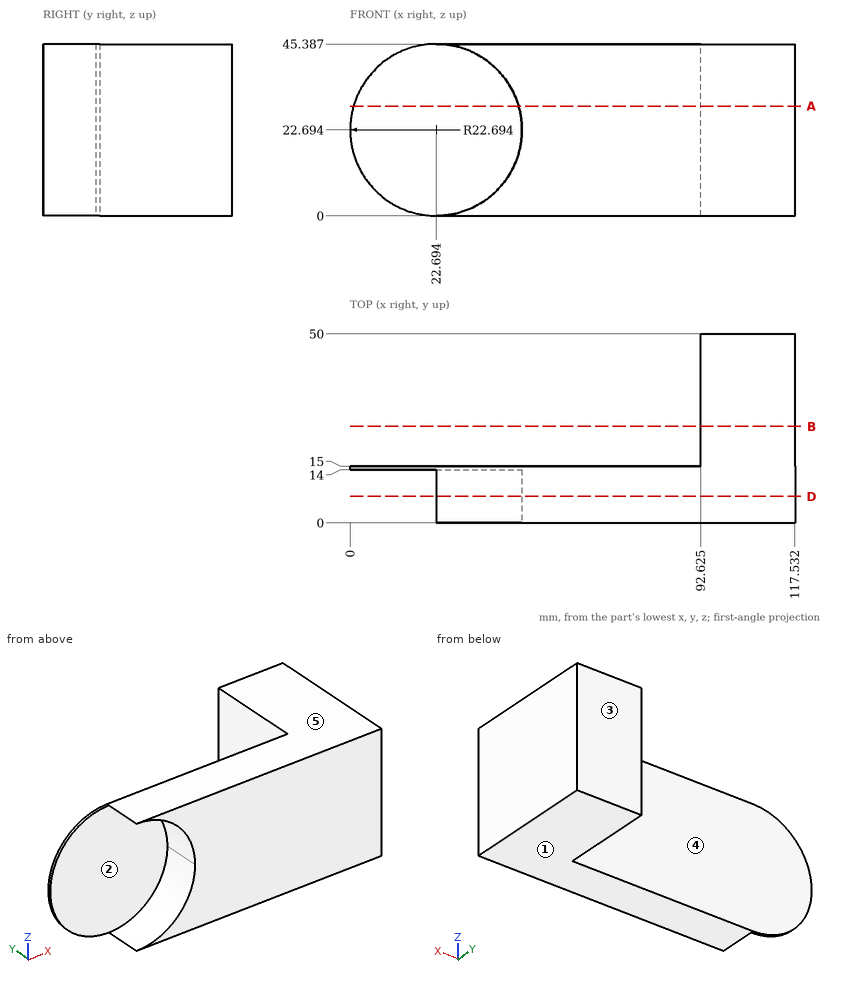
Here's the drawing with two shaded views (mm, measured from the low corner). I have some questions. A direction names the side the tool comes from. Round coordinates to 2 decimals unless told otherwise and drop trailing zeros. Order: outer loops, then holes, each group sorted by start corner. A loop starts at its lowest first (then second) coordinate and runs counter-clockwise, first axis right, second up. Notation, with made-up numbers: (29.5, 15) -> (62.5, 15) arc R20 ccw to (62.5, 20) -> close; hole circle Ø3 at (89, -26). An arc over 180 degrees is marked (long way). Return JSON: item names as keys, results as strings.
Q1. If we section it at B-B on y = 25.5: List the corners of the cut face in (x, z) for me (1 decimal), plus the area to 3 significant figures.
Filled sheet:
{"outline": "(92.6, 0) -> (117.5, 0) -> (117.5, 45.4) -> (92.6, 45.4) -> close", "area": "1,130 mm^2"}
Q2. For pin 1 Ø4 at (y, z) = (39.5, 18.5) entering from -X (3 decimals); pin 2 Ø4 at (x, z) = (44, 9.5) entering from +Y; pin 3 Ø22.5 at (x, z) = (24, 29) entering from -Y; pin 4 Ø6 at (x, y) = (89.5, 33) entering from -Z, each with a flat end and sliding along its axis, tell me the tip position at first contact or that it passes through.
Filled sheet:
{"pin 1": "stops at x = 92.625", "pin 2": "stops at y = 15", "pin 3": "stops at y = 14", "pin 4": "passes through"}
Q3. If we mould it in two halves opening along Z, with no side actions, what happens to the marked faces 1, 2 and 3? For each: released by +Z, released by -Z, zero draft, split by the parting line, or undercut.
Filled sheet:
{"face 1": "released by -Z", "face 2": "undercut", "face 3": "zero draft"}
Q4. I need wall thicknesses on line 1 along X through (y, z) = (40, 5) (1 decimal); line 2 along Y through (x, z) = (72, 32); line 3 along X through (y, z) = (13, 11.5) (1 decimal). Which ranges of each line are inside material? Lowest first, please. Write a range as from..to.
Filled sheet:
{"line 1": "x = 92.6..117.5", "line 2": "y = 0..15", "line 3": "x = 42.4..117.5"}
Q5. Which directions (+Z, -Z, +X, -X, +Y, -Y) give clear straight access to the entire face, cutting with the end or side of a thin tool? Please do the marked faces 4 and 5.
Filled sheet:
{"face 4": "+Z, -Z, -X, +Y", "face 5": "+Z, +X, -X, +Y, -Y"}
Q6. If we section it at A-A on z = 29: List the corners of the cut face in (x, y) for me (1 decimal), plus the area to 3 significant figures.
Filled sheet:
{"outline": "(0.9, 14) -> (44.5, 14) -> (44.5, 0) -> (117.5, 0) -> (117.5, 50) -> (92.6, 50) -> (92.6, 15) -> (0.9, 15) -> close", "area": "2,010 mm^2"}
Q7. If we section it at D-D on y = 7: List the corners of the cut face in (x, z) for me, plus the area to 3 significant figures.
Filled sheet:
{"outline": "(22.69, 0) -> (117.53, 0) -> (117.53, 45.39) -> (22.69, 45.39) arc R22.69 cw to start", "area": "3,500 mm^2"}
